Work out the finished part from the listing and answer in its coordinate system (mm). Coordinates: 2 decimals unless noted, no trailing zeros. Order: outer loops, then holes, each group sorted by start corner. A loop starts at its lowest first (then second) coordinate and runs counter-clockwise, first axis right, second up. Notation, with made-up numbers: M 84,51 L 135,51 A8 ccw 135,57 Z; hole C 84.25,75 d5. An arc over 180 degrees is marked long. Use a Markdown table: item, result.
from build123d import *

# Parameters (mm, degrees)
F0_W     = 17.734996
F0_H     = 17.848538
F1_DEPTH = 5.08
F2_W     = 114.3
F2_H     = 19.738256
F3_DEPTH = 7.62
F5_R     = 1.723631
F5_R_2   = 0.03756
F4_R     = 1.723627
F6_DEPTH = 3.81


with BuildPart() as f1:
    # F0 (on Top) → F1 (new body)
    with BuildSketch(Plane.XY):
        Rectangle(F0_W, F0_H)
    extrude(amount=F1_DEPTH)

    # F2 (on Top) → F3 (join)
    with BuildSketch(Plane.XY):
        Rectangle(F2_W, F2_H)
    extrude(amount=-F3_DEPTH)

    # F5 (on face) + F4 (on face) → F6 (join, symmetric)
    with BuildSketch(Plane(origin=(-57.15, 0, 0), x_dir=(0, -1, 0), z_dir=(-1, 0, 0))):
        with Locations((0, -3.627699)):
            Circle(F5_R)
        with Locations((0, -3.627699)):
            Circle(F5_R_2, mode=Mode.SUBTRACT)
    with BuildSketch(Plane.YZ.offset(57.15)):
        with Locations((0, -3.662557)):
            Circle(F4_R)
    extrude(amount=F6_DEPTH, both=True)


solid = f1.part
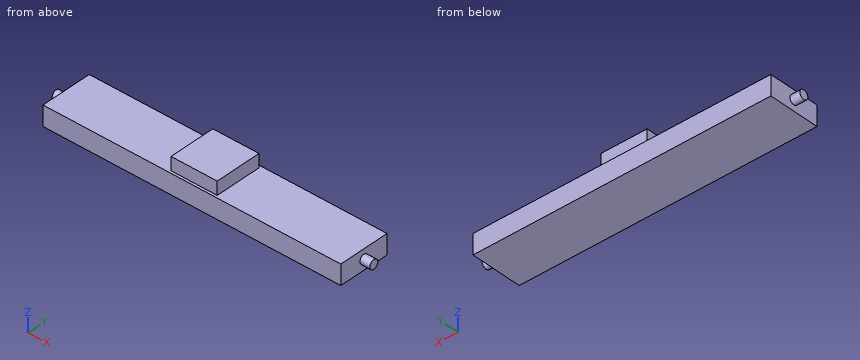
1. Find the intervals of material crossed by probe 1 along X at (y, z) = (8.75, -2.5); probe 2 along Z at (x, y) = (-44.5, -1.5); probe 3 along Y at (x, z) = (2, 2), in increasing order.
Answers below:
| item | result |
|---|---|
| probe 1 | -57.15 to 57.15 |
| probe 2 | -7.62 to 0 |
| probe 3 | -8.92 to 8.92 |
2. Flat-ended cylindrical pins translate along their axes: P1, Ø1, axis at y = 4.5, z = -1, coming from the +X side; P2, Ø4, axis at x = 3, z = 2.5, coming from the +Y side; P3, Ø5.5, axis at y = -2, z = 2, coming from the -X side. Find the tip coordinate at first contact, or state that the pin passes through.
Answers below:
| item | result |
|---|---|
| P1 | x = 57.15 |
| P2 | y = 8.92 |
| P3 | x = -57.15 |
3. Section C-C on z = 3.75 is taken. Determine the outline of the cut face in (x, y), then the cut area to 3 significant figures.
Answers below:
| item | result |
|---|---|
| outline | M -8.87,-8.92 L 8.87,-8.92 L 8.87,8.92 L -8.87,8.92 Z |
| area | 317 mm² |
4. Section B-B on x = -29 is taken. Determine the outline of the cut face in (y, z).
Answers below:
| item | result |
|---|---|
| outline | M -9.87,-7.62 L 9.87,-7.62 L 9.87,0 L -9.87,0 Z |
5. Section A-A on y = -5.25 is taken. Determine the outline of the cut face in (x, z).
Answers below:
| item | result |
|---|---|
| outline | M -57.15,-7.62 L 57.15,-7.62 L 57.15,0 L 8.87,0 L 8.87,5.08 L -8.87,5.08 L -8.87,0 L -57.15,0 Z |
